Here's how the part is built. I have some questions about the finished solid (model axes, mm). A direction names the side the tool comes from. Coordinates: 2 decimals unless noted, no trailing zeros. Write each loop counter-clockwise with the first axis right and the second up, starting at its lowest first coordinate (ties: lowest second). Pieces come first, ordered by that corner, then holes. Notation, with made-up numbers: (53.5, -21) -> (102.5, -21) arc R21 cw to (102.5, -16) -> close; hole circle Ø2 at (48.5, 21). An arc over 180 degrees is marked (long way). Put each result on its own line as item: value.
Autodesk Inventor part; units mm, degrees
ref_plane "Work Plane1" through (0, 0, -10) normal (0, 0, 1) x (1, 0, 0)
ref_plane "Work Plane3" through (0, 0, -28) normal (0, 0, 1) x (1, 0, 0)
ref_plane "YZ Plane" through (0, 0, 0) normal (1, 0, 0) x (0, 1, 0)
sketch "Sketch1" plane through (0, 0, 0) normal (0, 0, 1) x (1, 0, 0)
  circle A0 centre (0, 0) radius 12.5
  circle A1 centre (0, 0) radius 9
  circle A2 centre (0, 0) radius 11
  line L0 (17, -21) -> (-17, -21)
  line L1 (-21, -17) -> (-21, 17)
  line L2 (-17, 21) -> (17, 21)
  line L3 (21, 17) -> (21, -17)
  line L4 (21, -21) -> (-21, 21) construction
  line L5 (-21, -21) -> (21, 21) construction
  arc A3 (-17, 21) -> (-21, 17) centre (-17, 17) ccw
  arc A4 (-21, -17) -> (-17, -21) centre (-17, -17) ccw
  arc A5 (17, -21) -> (21, -17) centre (17, -17) ccw
  arc A6 (21, 17) -> (17, 21) centre (17, 17) ccw
  line L6 (15.5, -15.5) -> (-15.5, -15.5) construction
  line L7 (-15.5, -15.5) -> (-15.5, 15.5) construction
  line L8 (-15.5, 15.5) -> (15.5, 15.5) construction
  line L9 (15.5, 15.5) -> (15.5, -15.5) construction
  line L10 (15.5, -15.5) -> (-15.5, 15.5) construction
  line L11 (-15.5, -15.5) -> (15.5, 15.5) construction
  circle A7 centre (0, 0) radius 2.5
  circle A8 centre (0, 0) radius 4
  dimension "d0" = 42
  dimension "d2" = 42
  dimension "d3" = 4
  dimension "d4" = 18
  dimension "d5" = 22
  dimension "d6" = 25
  dimension "d7" = 31
  dimension "d22" = 5
  dimension "d23" = 8
ref_plane "Work Plane1" through (0, 0, -10) normal (0, 0, 1) x (1, 0, 0)
ref_plane "Work Plane3" through (0, 0, -28) normal (0, 0, 1) x (1, 0, 0)
ref_plane "Work Plane2" through (0, 0, -38) normal (0, 0, 1) x (1, 0, 0)
extrude "Extrusion1" add sketch "Sketch1" against normal up to surface (10 mm away) from surface at 0 contours A0 | A1 | A2 | L0 A4 L1 A3 L2 A6 L3 A5 | A7 | A8
sketch "Sketch2" plane through (17, 21, -10) normal (0, 0, -1) x (-1, 0, 0)
  arc A0 (34, -42) -> (38, -38) centre (34, -38) ccw
  line L0 (38, -38) -> (38, -4)
  arc A1 (38, -4) -> (34, 0) centre (34, -4) ccw
  line L1 (34, 0) -> (0, 0)
  arc A2 (0, 0) -> (-4, -4) centre (0, -4) ccw
  line L2 (-4, -4) -> (-4, -38)
  arc A3 (-4, -38) -> (0, -42) centre (0, -38) ccw
  line L3 (0, -42) -> (34, -42)
  line L4 (0, -0.1) -> (34, -0.1)
  arc A4 (37.9, -4) -> (34, -0.1) centre (34, -4) ccw
  line L5 (37.9, -4) -> (37.9, -38)
  arc A5 (34, -41.9) -> (37.9, -38) centre (34, -38) ccw
  line L6 (34, -41.9) -> (0, -41.9)
  arc A6 (-3.9, -38) -> (0, -41.9) centre (0, -38) ccw
  line L7 (-3.9, -38) -> (-3.9, -4)
  arc A7 (0, -0.1) -> (-3.9, -4) centre (0, -4) ccw
  point P0 (17, -21)
  dimension "d13" = 0.1
extrude "Extrusion2" add sketch "Sketch2" along normal up to surface (10 mm away) from surface at 18 contours L3 A3 L2 A2 L1 A1 L0 A0 | L4 A4 L5 A5 L6 A6 L7 A7
extrude "Extrusion3" add sketch "Sketch2" along normal up to surface (18 mm away) from surface at 0 contours L4 A4 L5 A5 L6 A6 L7 A7
extrude "Extrusion4" cut sketch "Sketch1" against normal blind 0.5 contours A0 | A1 | A8
extrude "Extrusion5" add sketch "Sketch1" along normal blind 2 contours A2
extrude "Extrusion6" cut sketch "Sketch1" against normal blind 2 contours A8
extrude "Extrusion7" add sketch "Sketch1" along normal blind 25 contours A7
hole "Hole1" at (15.5, 15.5, 0) at (-15.5, 15.5, 0) at (-15.5, -15.5, 0) at (15.5, -15.5, 0) direction (0, 0, -1) diameter 2.459 depth 4 tip angle 118
sketch "Sketch3" plane through (21, -17, -38) normal (1, 0, 0) x (0, 0, -1)
  line L0 (0, 34) -> (0, 0)
  line L1 (-10, 34) -> (-10, 0)
  line L2 (-10, 17) -> (0, 17) construction
  line L3 (-9.9, 9.5) -> (-3.9, 9.5)
  line L4 (-3.9, 9.5) -> (-3.9, 24.5)
  line L5 (-3.9, 24.5) -> (-9.9, 24.5)
  line L6 (-9.9, 24.5) -> (-9.9, 9.5)
  line L7 (-9.9, 9.5) -> (-3.9, 24.5) construction
  line L8 (-3.9, 9.5) -> (-9.9, 24.5) construction
  line L9 (-9.8, 8.5) -> (-0.8, 8.5)
  line L10 (-0.8, 8.5) -> (-0.8, 25.5)
  line L11 (-0.8, 25.5) -> (-9.8, 25.5)
  line L12 (-9.8, 25.5) -> (-9.8, 8.5)
  line L13 (-9.8, 8.5) -> (-0.8, 25.5) construction
  line L14 (-0.8, 8.5) -> (-9.8, 25.5) construction
  point P0 (-38, 17)
  point P1 (-6.9, 17)
  point P2 (-5.3, 17)
  dimension "d35" = 6
  dimension "d36" = 15
  dimension "d37" = 9
  dimension "d38" = 17
  dimension "d39" = 0.1
  dimension "d40" = 0.1
extrude "Extrusion8" add sketch "Sketch3" along normal blind 6 contours L6 L5 L12 L3 | L12 L5 L4 L3
extrude "Extrusion9" add sketch "Sketch3" along normal blind 1.5 contours L12 L5 L4 L3 | L3 L4 L5 L12 L11 L10 L9
equation "\"d9\" = -L"
equation "\"L\" = 38"
properties part number "nema17 33mm"
Item 1: For P1, Ø14.5, axis at y = 5.5, z = -21, coming from the -X side; P2, Ø1.5, axis at y = 9.5, z = 1.5, coming from the -X side; P3, Ø1.8, axis at x = 23.5, z = -30, coming from the +Y side; P4, Ø12.5, axis at x = 4, y = -9, coming from the +Z side, each with a flat end and sliding along its axis, tell me the tip position at first contact or that it passes through.
Output:
P1: stops at x = -21
P2: stops at x = -6.67
P3: stops at y = 7.5
P4: stops at z = 2
Item 2: Please list where these lines run through material, in increasing order: line 1 along Y through (x, z) = (0, -0.05); line 2 along Y through (x, z) = (-15.5, -3). Write a range as from..to.
Output:
line 1: y = -21..-12.5, -11..-9, -2.5..2.5, 9..11, 12.5..21
line 2: y = -21..-16.73, -14.27..14.27, 16.73..21
Item 3: If we mould it in two halves opening along X, with no side actions, what happens to faces 1 (the flat face through (0, -20.9, -19)), 2 (the conical face through (15.64, -15.34, -4.61)), 3 (the cylindrical face through (15.131, -16.673, -2.028)), 4 (the cylindrical face through (-19.788, -19.727, -18.874))? For each: released by +X, released by -X, zero draft, split by the parting line, or undercut.
Output:
face 1: zero draft
face 2: undercut
face 3: undercut
face 4: released by -X
Item 4: Which directions (+Z, -Z, +X, -X, +Y, -Y) give clear straight access to the entire face, cutting with the end or side of a thin tool? Please do faces 5 (the flat face through (22, 8.5, -33)), 6 (the cylindrical face through (-0.867, -3.905, -1.24)), 7 (the flat face through (21, 0, -5)).
Output:
face 5: +Z, -Z, +X, +Y
face 6: +Z
face 7: +Z, +X, +Y, -Y
Item 5: Imagine slicing it at B-B on z = -12. Write out the boundary of the cut face in (x, y).
Output:
outline: (-20.9, -17) arc R3.9 ccw to (-17, -20.9) -> (17, -20.9) arc R3.9 ccw to (20.9, -17) -> (20.9, 17) arc R3.9 ccw to (17, 20.9) -> (-17, 20.9) arc R3.9 ccw to (-20.9, 17) -> close
Item 6: Imagine slicing it at A-A on x = -13.5. Write out the boundary of the cut face in (y, z).
Output:
outline: (-21, -38) -> (21, -38) -> (21, -28) -> (20.9, -28) -> (20.9, -10) -> (21, -10) -> (21, 0) -> (-21, 0) -> (-21, -10) -> (-20.9, -10) -> (-20.9, -28) -> (-21, -28) -> close
Item 7: Imagine slicing it at D-D on z = 5.5. Write out the boundary of the cut face in (x, y).
Output:
outline: circle Ø5 at (0, 0)
